from build123d import *

# Parameters (mm, degrees)
F0_R     = 3.302
F1_DEPTH = 2.54
F3_DEPTH = 2.54
F4_W     = 6.096
F4_H     = 19.05
F5_DEPTH = 2.54
F6_R     = 0.635
F7_W     = 2.286
F7_H     = 10.668
F8_DEPTH = 25.4


with BuildPart() as f1:
    # F0 (on Top) → F1 (new body)
    with BuildSketch(Plane.XY):
        Circle(F0_R)
    extrude(amount=F1_DEPTH)

    # F2 (on face) → F3 (join, through all)
    with BuildSketch(Plane(origin=(0, 0, 0), x_dir=(1, 0, 0), z_dir=(0, 0, -1))):
        with BuildLine():
            ThreePointArc((2.2225, -2.442068), (0, -3.302), (-2.2225, -2.442068))
            Line((-2.2225, -2.442068), (-2.2225, -4.474068))
            Line((-2.2225, -4.474068), (2.2225, -4.474068))
            Line((2.2225, -4.474068), (2.2225, -2.442068))
        make_face()
    extrude(amount=-F3_DEPTH)

    # F4 (on Top) → F5 (join, through all)
    with BuildSketch(Plane.XY):
        with Locations((0, 13.999068)):
            Rectangle(F4_W, F4_H)
    extrude(amount=F5_DEPTH)

    # F6
    f6_edges = [f1.edges().sort_by_distance(p)[0] for p in [
        (3.048, 4.474068, 1.27),
        (-3.048, 4.474068, 1.27),
    ]]
    fillet(f6_edges, radius=F6_R)

    # F7 (on face) → F8 (cut)
    with BuildSketch(Plane.XY.offset(2.54)):
        with Locations((0, 12.7)):
            Rectangle(F7_W, F7_H)
    extrude(amount=-F8_DEPTH, mode=Mode.SUBTRACT)

    # F9: F1 across face


with BuildPart() as f1_1:
    add(f1.part)
    add(f1.part.mirror(Plane(origin=(0, 23.524068, 1.27), x_dir=(-1, 0, 0), z_dir=(0, 1, 0))))


solid = f1_1.part
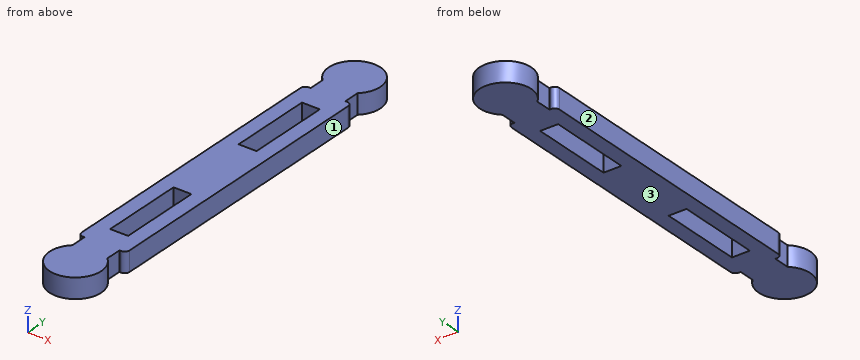
The listing builds one solid part. Answer for the finished solid, in the listing's coordinates (mm). Face numbers are marked on the shaded views. A direction names the side the tool comes from. Give positions to 0.01 mm unless a question says otherwise; leave off trailing zeros. Loops run counter-clockwise (first coordinate to the right, second up) from the corner with the lowest first, then second, coordinate; pieces in that order, holes last. Notation, with made-up numbers: M 37,34.5 L 72,34.5 A18 cw 72,47.5 Z; hole C -31.75,-27.5 d6. An arc over 180 degrees is marked long. Answer as CSV lines item,"result".
Item 1: The part is cut by section B-B (x = 0). Give the vertices of the cut face in (y, z).
Values follow:
outline,"M -3.3,0 L 7.37,0 L 7.37,2.54 L -3.3,2.54 Z; M 18.03,0 L 29.01,0 L 29.01,2.54 L 18.03,2.54 Z; M 39.68,0 L 50.35,0 L 50.35,2.54 L 39.68,2.54 Z"
Item 2: Given pin 1 Ø0.8 at (y, z) = (12.5, 2) entering from +X; pin 2 Ø0.6 at (y, z) = (43.5, 2) entering from -X; pin 3 Ø1.3 at (y, z) = (13, 1) entering from -X, each flat-ended and moving along its own axis, determine where each tip first touches the part or whether it passes through.
Values follow:
pin 1,"stops at x = 3.05"
pin 2,"stops at x = -2.22"
pin 3,"stops at x = -3.05"
Item 3: The part is cut by section D-D (y = 44). Give the vertices of the cut face in (x, z).
Values follow:
outline,"M -2.22,0 L 2.22,0 L 2.22,2.54 L -2.22,2.54 Z"
Item 4: The part is cut by section A-A (z = 1.7). Give the number of separate pieces and of enclosed holes in the cut face, and give its area (3 significant figures).
Values follow:
separate pieces,"1"
enclosed holes,"2"
area,"264 mm^2"
Item 5: Straight lines are drawn through the part: line 1 along Y through (x, z) = (0, 2.3); line 2 along X through (y, z) = (8.5, 0.35); line 3 along Y through (x, z) = (-1, 1.8). For each, find the intervals that lie inside material, in ascending order. Write a range as [from, to].
Values follow:
line 1,"y = [-3.3, 7.37], [18.03, 29.01], [39.68, 50.35]"
line 2,"x = [-3.05, -1.14], [1.14, 3.05]"
line 3,"y = [-3.15, 7.37], [18.03, 29.01], [39.68, 50.2]"
Item 6: The part is cut by section C-C (y = 13.5). Give the vertices of the cut face in (x, z).
Values follow:
outline,"M -3.05,0 L -1.14,0 L -1.14,2.54 L -3.05,2.54 Z; M 1.14,0 L 3.05,0 L 3.05,2.54 L 1.14,2.54 Z"
Item 7: Which of the six approach directions +Z, -Z, +X, -X, +Y, -Y give full straight-line access (tool end or side, diameter ignored) to the marked faces 1, 2 and 3?
Values follow:
face 1,"+Z, -Z, +X"
face 2,"+Z, -Z, -X"
face 3,"-Z, +X, -X, +Y, -Y"
